from build123d import *

# Parameters (mm, degrees)
SKETCH1_W           = 15
SKETCH1_H           = 15
SKETCH1_R           = 3.302
BOSS_EXTRUDE1_DEPTH = 3
SKETCH2_W           = 15
SKETCH2_H           = 18
SKETCH2_R           = 1.5
BOSS_EXTRUDE2_DEPTH = 3
BOSS_EXTRUDE3_DEPTH = 3


with BuildPart() as part:
    # Sketch1 → Boss-Extrude1 (new body)
    with BuildSketch(Plane.XY):
        Rectangle(SKETCH1_W, SKETCH1_H)
        Circle(SKETCH1_R, mode=Mode.SUBTRACT)
    extrude(amount=BOSS_EXTRUDE1_DEPTH)

    # Sketch2 → Boss-Extrude2 (add)
    with BuildSketch(Plane.XZ.offset(7.5)):
        with Locations((0, 9)):
            Rectangle(SKETCH2_W, SKETCH2_H)
        with Locations((0, 10.5)):
            Circle(SKETCH2_R, mode=Mode.SUBTRACT)
    extrude(amount=BOSS_EXTRUDE2_DEPTH)

    # Sketch3 → Boss-Extrude3 (add)
    with BuildSketch(Plane(origin=(7.5, 0, 0), x_dir=(0, 0, -1), z_dir=(1, 0, 0))):
        Polygon((-18, -10.5), (-18, -7.5), (-3, 7.5), (0, 7.5), (0, -10.5), align=None)
    boss_extrude3 = extrude(amount=BOSS_EXTRUDE3_DEPTH)

    # Mirror1: Boss-Extrude3 across plane
    add(boss_extrude3.mirror(Plane(origin=(0, 0, 0), x_dir=(0, 0, 1), z_dir=(1, 0, 0))))


solid = part.part
Work out the finished part from the listing and answer in its coordinate system (mm). A direction names the side the tool comes from. Round coordinates to 2 decimals unless told otherwise and drop trailing zeros. Loops run counter-clockwise (first coordinate to the right, second up) from the corner with the lowest first, then second, coordinate; pieces in that order, holes last. Notation, with made-up numbers: (73.25, 86.5) -> (90.25, 86.5) arc R19 cw to (90.25, 99.5) -> close; hole circle Ø8 at (-31.75, -22.5). An arc over 180 degrees is marked (long way). Use one line per item in the form item = value.
(1) For a pull along Z with two mould halves and no side action, classify faces 1 (the flat face through (-2, 3, 3)), 2 (the cylindrical face through (0, -9, 9)), 3 (the flat face through (0, -10.5, 7)) as released by +Z, released by -Z, zero draft, split by the parting line, or undercut.
Answer list:
face_1 = released by +Z
face_2 = undercut
face_3 = zero draft
(2) Flat-ended cylindrical pins translate along their axes: P1, Ø1, axis at x = 7.5, y = 4.5, coming from the +Z side; P2, Ø6, axis at x = 0, y = 0, coming from the -Z side; P3, Ø2, axis at x = -0.5, y = -4.5, coming from the -Z side; P4, Ø7.5, axis at x = -1.5, y = 0.5, coming from the +Z side. Find the tip coordinate at first contact, or state that the pin passes through.
Answer list:
P1 = 6.5
P2 = through
P3 = 0
P4 = 3
(3) Find section C-C on y = 0. Give the vertices of the cut face in (x, z).
Answer list:
outline = (-10.5, 0) -> (-3.3, 0) -> (-3.3, 3) -> (-7.5, 3) -> (-7.5, 10.5) -> (-10.5, 10.5) -> close; (3.3, 0) -> (10.5, 0) -> (10.5, 10.5) -> (7.5, 10.5) -> (7.5, 3) -> (3.3, 3) -> close
(4) A tool of negligible diameter and unlimited length cuts with its end or side. For faces 4 (the flat face through (9, -0.1, 10.6)), 5 (the flat face through (-0.1, -7.5, 12.3)), from which of +Z, -Z, +X, -X, +Y, -Y can it reach the whole face along a straight path? Write none if from no direction.
Answer list:
face_4 = +Z, +X, -X, +Y
face_5 = +Z, +Y
(5) Find section B-B on z = 10.5. Give the vertices of the cut face in (x, y).
Answer list:
outline = (-10.5, -10.5) -> (-1.5, -10.5) -> (-1.5, -7.5) -> (-7.5, -7.5) -> (-7.5, 0) -> (-10.5, 0) -> close; (1.5, -10.5) -> (10.5, -10.5) -> (10.5, 0) -> (7.5, 0) -> (7.5, -7.5) -> (1.5, -7.5) -> close
(6) Find section A-A on x = 0. Give the vertices of the cut face in (y, z), then the cut area to 3 significant figures.
Answer list:
outline = (-10.5, 0) -> (-3.3, 0) -> (-3.3, 3) -> (-7.5, 3) -> (-7.5, 9) -> (-10.5, 9) -> close; (-10.5, 12) -> (-7.5, 12) -> (-7.5, 18) -> (-10.5, 18) -> close; (3.3, 0) -> (7.5, 0) -> (7.5, 3) -> (3.3, 3) -> close
area = 70.2 mm2
(7) Find section D-D on z = 14.5. Give the vertices of the cut face in (x, y), then the cut area to 3 significant figures.
Answer list:
outline = (-10.5, -10.5) -> (10.5, -10.5) -> (10.5, -4) -> (7.5, -4) -> (7.5, -7.5) -> (-7.5, -7.5) -> (-7.5, -4) -> (-10.5, -4) -> close
area = 84.0 mm2
(8) Straight lines are drawn through the part: line 1 (X direction, y = 1, z = 8); line 2 (Z direction, x = -6.5, y = 0.5); line 3 (Z direction, x = 0, y = -8.5). For each, find the intervals that lie inside material, in ascending order.
Answer list:
line_1 = -10.5 to -7.5, 7.5 to 10.5
line_2 = 0 to 3
line_3 = 0 to 9, 12 to 18
